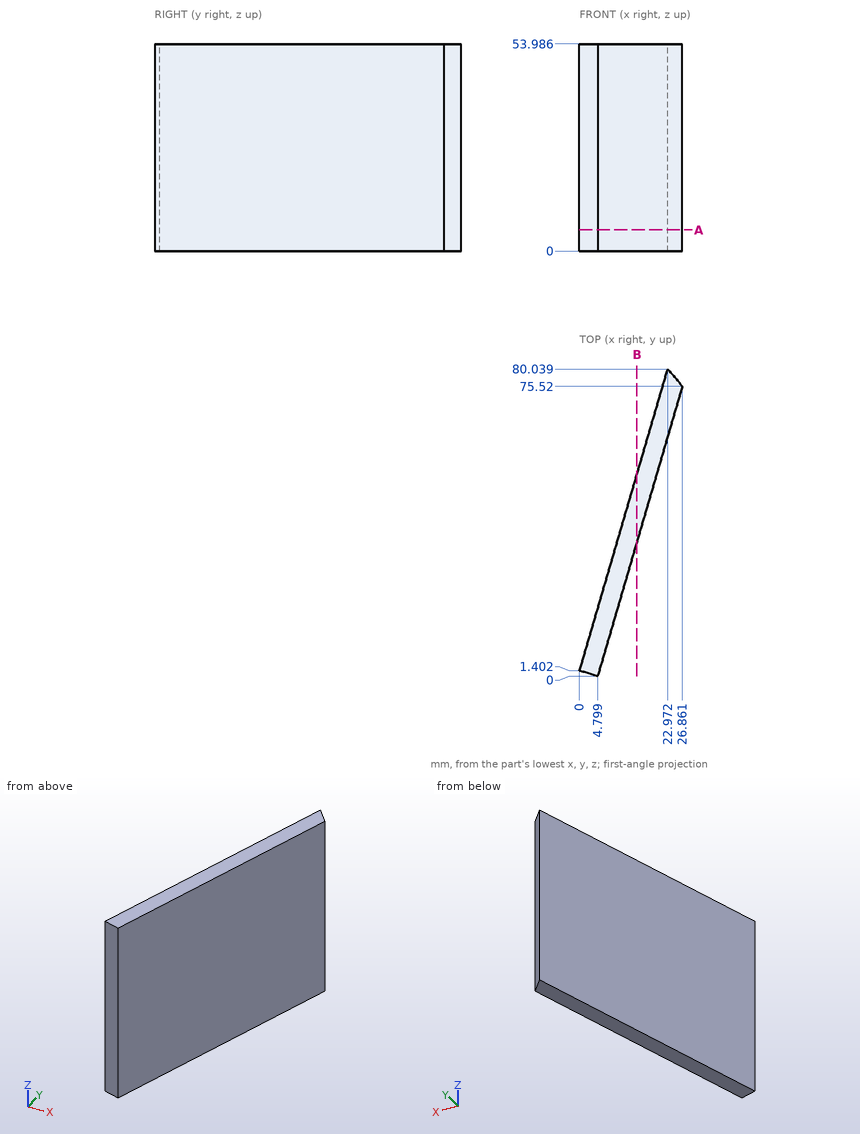
Design review of the part shown in the three views and the two pictorial views. Dimensions are in mm from the part's minimum x, y and z. Round coordinates to 2 decimals unless told otherwise and drop trailing zeros. Loops run counter-clockwise (first coordinate to the right, second up) from the corner with the lowest first, then second, coordinate; pieces in that order, holes last. Notation, with made-up numbers: (-27, 27) -> (-21, 27) arc R36 ccw to (-21, 65) -> close; hole circle Ø7 at (86.5, -35). An arc over 180 degrees is marked (long way). Answer as a JSON object with one key per item and string values. Group by question number.
1) We need section A-A on z = 5.5. Write out the cut boundary in (x, y).
2) For line 1 (X direction, y = 6, z = 45); line 2 (X direction, y = 26.5, z = 35), list the stretches that pass through material, from the lowest coordinate up. Write a range as [from, to].
3) For pin 1 Ø1 at (y, z) = (48, 38.5) entering from -X; pin 2 Ø1.5 at (y, z) = (46.5, 13.5) entering from -X (1 decimal); pin 3 Ø3 at (y, z) = (61.5, 34) entering from -X, all flat-tipped, find the tip position at first contact; note any pin that passes through.
4) We need section B-B on x = 15. Write out the cut boundary in (y, z).
Result set:
{
 "1": {"outline": "(0, 1.4) -> (4.8, 0) -> (26.86, 75.52) -> (22.97, 80.04) -> close"},
 "2": {"line 1": "[1.34, 6.55]", "line 2": "[7.33, 12.54]"},
 "3": {"pin 1": "x = 13.47", "pin 2": "x = 13", "pin 3": "x = 17.12"},
 "4": {"outline": "(34.92, 0) -> (52.75, 0) -> (52.75, 53.99) -> (34.92, 53.99) -> close"}
}
